Verification items for the finished model (mm, model axes). Round coordinates to 2 decimals unless told otherwise and drop trailing zeros. Loops run counter-clockwise (first coordinate to the right, second up) from the corner with the lowest first, then second, coordinate; pieces in that order, holes last. Notation, with made-up numbers: M -35,43 L -14,43 A17 cw -14,60 Z; hole C -26,45 d4. An arc over 180 degrees is marked long. Answer as CSV lines item,"result".
```python
from build123d import *

# Parameters (mm, degrees)
F0_W     = 50
F0_H     = 140
F1_DEPTH = 5
F3_D     = 4
F6_DEPTH = 25
F7_R     = 15.526878
F8_R     = 9.599373


with BuildPart() as f1:
    # F0 (on Top) → F1 (new body)
    with BuildSketch(Plane.XY):
        with Locations((25, 70)):
            Rectangle(F0_W, F0_H)
    extrude(amount=F1_DEPTH)

    # F3 (through all)
    with Locations(Plane.XY.offset(5)):
        with Locations((25, 30), (25, 80)):
            Hole(F3_D / 2)

    # F5 (on face) → F6 (cut)
    with BuildSketch(Plane.XY.offset(5)):
        with BuildLine():
            ThreePointArc((37, 30), (40, 27), (43, 30))
            Line((43, 30), (43, 80))
            ThreePointArc((43, 80), (40, 83), (37, 80))
            Line((37, 80), (37, 30))
        make_face()
    extrude(amount=-F6_DEPTH, mode=Mode.SUBTRACT)

    # F7
    f7_edges = [f1.edges().sort_by_distance(p)[0] for p in [
        (50, 140, 2.5),
    ]]
    fillet(f7_edges, radius=F7_R)

    # F8
    f8_edges = [f1.edges().sort_by_distance(p)[0] for p in [
        (50, 0, 2.5),
    ]]
    fillet(f8_edges, radius=F8_R)

    # F9: F1 across plane


with BuildPart() as f1_1:
    add(f1.part)
    add(f1.part.mirror(Plane.YZ))


solid = f1_1.part
```
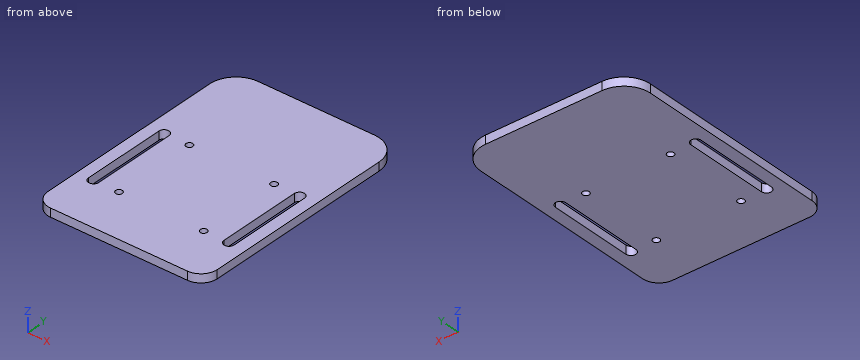
1) Material ranges on probe 1 along X at (y, z) = (38, 1.25); probe 2 along Y at (x, z) = (25, 3.15); probe 3 along X at (y, z) = (29, 0.8), recorded low to high.
Here are the results:
probe 1,"x = -50 to -43, -37 to 37, 43 to 50"
probe 2,"y = 0 to 28, 32 to 78, 82 to 140"
probe 3,"x = -50 to -42.83, -37.17 to -26.73, -23.27 to 23.27, 26.73 to 37.17, 42.83 to 50"
2) Section check B-B (z = 2.6). Record the cut outline in (x, y), plus the area to 3 significant figures.
Here are the results:
outline,"M -50,9.6 A9.6 ccw -40.4,0 L 40.4,0 A9.6 ccw 50,9.6 L 50,124.47 A15.53 ccw 34.47,140 L -34.47,140 A15.53 ccw -50,124.47 Z; hole M -43,30 A3 ccw -37,30 L -37,80 A3 ccw -43,80 Z; hole C -25,30 d4; hole C -25,80 d4; hole C 25,30 d4; hole C 25,80 d4; hole M 37,30 A3 ccw 43,30 L 43,80 A3 ccw 37,80 Z"
area,"13,200 mm^2"
3) Section check C-C (x = -25). Record the cut outline in (y, z).
Here are the results:
outline,"M 0,0 L 28,0 L 28,5 L 0,5 Z; M 32,0 L 78,0 L 78,5 L 32,5 Z; M 82,0 L 140,0 L 140,5 L 82,5 Z"
4) Section check A-A (y = 40.5). Record the cut outline in (x, z).
Here are the results:
outline,"M -50,0 L -43,0 L -43,5 L -50,5 Z; M -37,0 L 37,0 L 37,5 L -37,5 Z; M 43,0 L 50,0 L 50,5 L 43,5 Z"
